Source: CAD feature listing. Evaluate the final solid. Frame: model axes, mm. Round coordinates to 2 decimals unless told otherwise and drop trailing zeros. Loops run counter-clockwise (first coordinate to the right, second up) from the corner with the lowest first, then second, coordinate; pieces in that order, holes last.
Item 1: Section query A-A on y = 48. Return loops of the section in (x, z).
Item 2: Section query C-C on y = 59. Return loops of the section in (x, z).
Item 3: Section query B-B on z = 82. Return loops of the section in (x, y), then the cut area to 3 significant figures.
Item 4: Ray query, L1, parallel to Z at x = 84.05, y = 57; L2, parallel to Z at x = 87.8, y = 53.25; L3, parallel to Z at x = 86.5, y = 52. Return the intervals inside material, ascending.
Item 5: First-contact query: P1, Ø3, axis at x = 85, z = 49.5, coming from the +Y side; P2, Ø1, axis at x = 85, y = 57, coming from the +Z side; P3, Ø2, axis at x = 87, y = 55.5, coming from the -Z side; P4, Ø6, axis at y = 51, z = 69.5, coming from the -X side. Flat tips, straight axial feed; report the tip coordinate or a pass-through.
```python
from build123d import *

# Parameters (mm, degrees)
SKETCH1_W           = 5
SKETCH1_H           = 11
BOSS_EXTRUDE1_DEPTH = 150
CUT_EXTRUDE1_DEPTH  = 161.573187019
SKETCH3_W           = 5
SKETCH3_H           = 30
BOSS_EXTRUDE2_DEPTH = 5
CUT_EXTRUDE2_DEPTH  = 163.417988138
SKETCH6_W           = 5
SKETCH6_H           = 8
BOSS_EXTRUDE3_DEPTH = 3
SKETCH7_W           = 5
SKETCH7_H           = 8
BOSS_EXTRUDE4_DEPTH = 3
SKETCH8_W           = 5
SKETCH8_H           = 5
CUT_EXTRUDE3_DEPTH  = 166.192623536


with BuildPart() as part:
    # Sketch1 → Boss-Extrude1 (new body)
    with BuildSketch(Plane.XY):
        with Locations((85.894042166, 51.58544814)):
            Rectangle(SKETCH1_W, SKETCH1_H)
    extrude(amount=BOSS_EXTRUDE1_DEPTH)

    # Sketch2 → Cut-Extrude1 (cut, through all)
    with BuildSketch(Plane(origin=(88.394042166, 0, 0), x_dir=(0, 0, -1), z_dir=(1, 0, 0))):
        with BuildLine():
            Line((-93, 53.08544814), (-57, 53.08544814))
            ThreePointArc((-57, 53.08544814), (-52.050252532, 51.035195608), (-50, 46.08544814))
            Line((-50, 46.08544814), (-100, 46.08544814))
            ThreePointArc((-100, 46.08544814), (-97.949747468, 51.035195608), (-93, 53.08544814))
        make_face()
    extrude(amount=-CUT_EXTRUDE1_DEPTH, mode=Mode.SUBTRACT)

    # Sketch3 → Boss-Extrude2 (add)
    with BuildSketch(Plane(origin=(0, 57.08544814, 0), x_dir=(1, 0, 0), z_dir=(0, 1, 0))):
        with Locations((85.894042166, -75)):
            Rectangle(SKETCH3_W, SKETCH3_H)
    extrude(amount=BOSS_EXTRUDE2_DEPTH)

    # Sketch5 → Cut-Extrude2 (cut, through all)
    with BuildSketch(Plane(origin=(88.394042166, 0, 0), x_dir=(0, 0, -1), z_dir=(1, 0, 0))):
        Polygon((-35.5, 55.08544814), (-34.25, 55.08544814), (-34.25, 52.53544814), (-35.5, 52.53544814), (-35.5, 51.08544814), (-38.5, 51.08544814), (-38.5, 52.53544814), (-39.75, 52.53544814), (-39.75, 55.08544814), (-38.5, 55.08544814), (-38.5, 57.08544814), (-35.5, 57.08544814), align=None)
        Polygon((-114.5, 52.53544814), (-115.75, 52.53544814), (-115.75, 55.08544814), (-114.5, 55.08544814), (-114.5, 57.08544814), (-111.5, 57.08544814), (-111.5, 55.08544814), (-110.25, 55.08544814), (-110.25, 52.53544814), (-111.5, 52.53544814), (-111.5, 51.08544814), (-114.5, 51.08544814), align=None)
    extrude(amount=-CUT_EXTRUDE2_DEPTH, mode=Mode.SUBTRACT)

    # Sketch6 → Boss-Extrude3 (add)
    with BuildSketch(Plane(origin=(0, 0, 0), x_dir=(-1, 0, 0), z_dir=(0, 0, -1))):
        with Locations((-85.894042166, 50.08544814)):
            Rectangle(SKETCH6_W, SKETCH6_H)
    extrude(amount=BOSS_EXTRUDE3_DEPTH)

    # Sketch7 → Boss-Extrude4 (add)
    with BuildSketch(Plane.XY.offset(150)):
        with Locations((85.894042166, 50.08544814)):
            Rectangle(SKETCH7_W, SKETCH7_H)
    extrude(amount=BOSS_EXTRUDE4_DEPTH)

    # Sketch8 → Cut-Extrude3 (cut, through all)
    with BuildSketch(Plane(origin=(88.394042166, 0, 0), x_dir=(0, 0, -1), z_dir=(1, 0, 0))):
        with Locations((-123.5, 54.58544814)):
            Rectangle(SKETCH8_W, SKETCH8_H)
        with Locations((-26.5, 54.58544814)):
            Rectangle(SKETCH8_W, SKETCH8_H)
    extrude(amount=-CUT_EXTRUDE3_DEPTH, mode=Mode.SUBTRACT)


solid = part.part
```
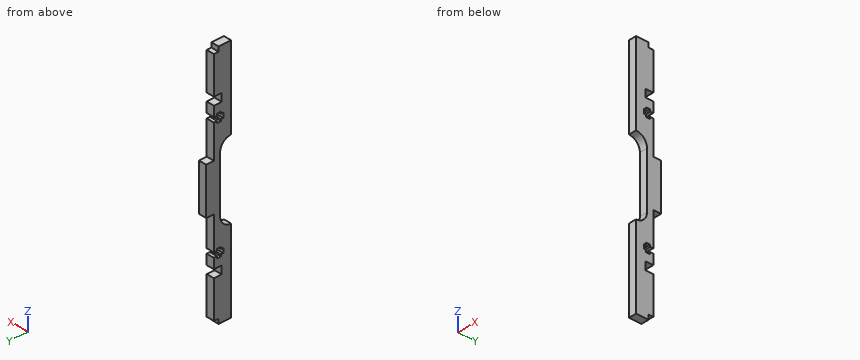
Data:
1. outline: (83.39, -3) - (88.39, -3) - (88.39, 50.27) - (83.39, 50.27) - close; (83.39, 99.73) - (88.39, 99.73) - (88.39, 153) - (83.39, 153) - close
2. outline: (83.39, 60) - (88.39, 60) - (88.39, 90) - (83.39, 90) - close
3. outline: (83.39, 53.09) - (88.39, 53.09) - (88.39, 62.09) - (83.39, 62.09) - close
3. area: 45.0 mm2
4. L1: z = 0 to 24, 29 to 35.5, 38.5 to 111.5, 114.5 to 121, 126 to 150
4. L2: z = -3 to 24, 29 to 34.25, 39.75 to 110.25, 115.75 to 121, 126 to 153
4. L3: z = -3 to 35.5, 38.5 to 53.26, 96.74 to 111.5, 114.5 to 153
5. P1: stops at y = 57.09
5. P2: stops at z = 150
5. P3: stops at z = 0
5. P4: stops at x = 83.39
